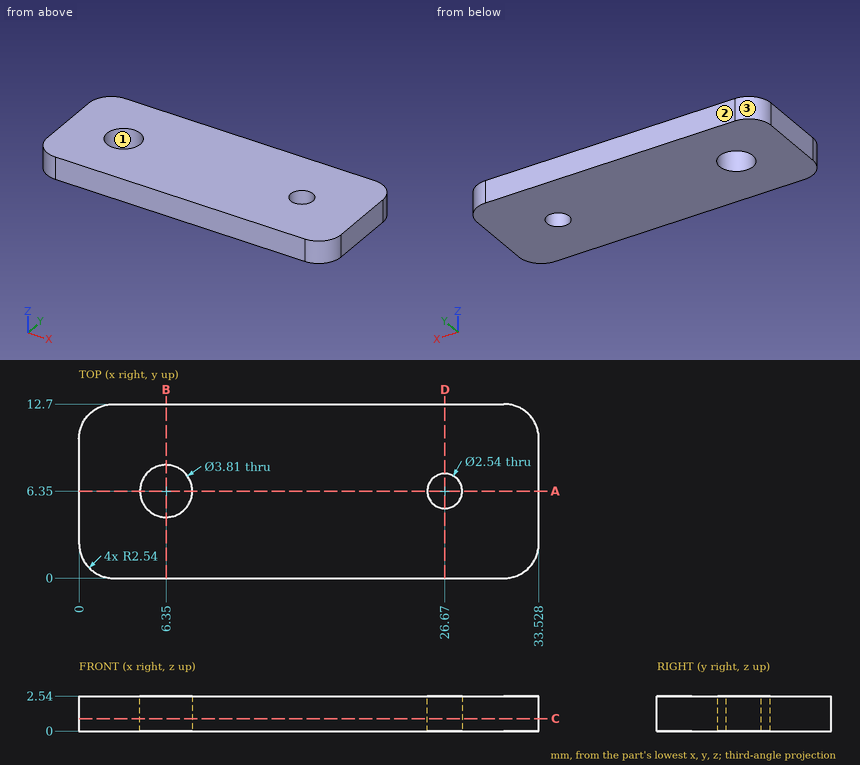
Print and shaded views of the part. All mm, measured from the part's lowest x, y and z. Round coordinates to 2 decimals unless told otherwise and drop trailing zeros. Write each loop counter-clockwise with the first axis right and the second up, starting at its lowest first coordinate (ties: lowest second). Pieces come first, ordered by that corner, then holes.
Item 1: Cut at D-D, the plane x = 26.67. Give the cut face in (y, z).
Results:
outline: (0, 0) - (5.08, 0) - (5.08, 2.54) - (0, 2.54) - close; (7.62, 0) - (12.7, 0) - (12.7, 2.54) - (7.62, 2.54) - close
Item 2: Cut at A-A, the plane y = 6.35. Give the cut face in (x, z) (3 decimals).
Results:
outline: (0, 0) - (4.445, 0) - (4.445, 2.54) - (0, 2.54) - close; (8.255, 0) - (25.4, 0) - (25.4, 2.54) - (8.255, 2.54) - close; (27.94, 0) - (33.528, 0) - (33.528, 2.54) - (27.94, 2.54) - close
Item 3: Cut at B-B, the plane x = 6.35. Give the cut face in (y, z) (3 decimals).
Results:
outline: (0, 0) - (4.445, 0) - (4.445, 2.54) - (0, 2.54) - close; (8.255, 0) - (12.7, 0) - (12.7, 2.54) - (8.255, 2.54) - close
Item 4: Probe L1, parallel to Y at x = 6.35, z = 0.95 (3 decimals); L2, parallel to X at y = 7, z = 2.45; L3, parallel to X at y = 7.75, z = 1.3. List the from-to ranges inside material, lowest first.
Results:
L1: y = 0 to 4.445, 8.255 to 12.7
L2: x = 0 to 4.56, 8.14 to 25.58, 27.76 to 33.53
L3: x = 0 to 5.06, 7.64 to 33.53
Item 5: Drop flat-ended pins along their axis: pin 1 Ø6 at (x, y) = (26, 6) entering from +Z; pin 2 Ø1.5 at (x, y) = (26.67, 6.35) entering from +Z. Give the stop position or say it passes through.
Results:
pin 1: stops at z = 2.54
pin 2: passes through
Item 6: Cut at C-C, the plane z = 0.9. Give the cut face in (x, y) (3 decimals).
Results:
outline: (0, 2.54) arc R2.54 ccw to (2.54, 0) - (30.988, 0) arc R2.54 ccw to (33.528, 2.54) - (33.528, 10.16) arc R2.54 ccw to (30.988, 12.7) - (2.54, 12.7) arc R2.54 ccw to (0, 10.16) - close; hole circle Ø3.81 at (6.35, 6.35); hole circle Ø2.54 at (26.67, 6.35)
Item 7: Two-plate mould, pull along X, no slides. Class the marked faces 1, 2 and 3: +X half, -X half, draft (parallel to the pull), parting line (faces both ways), or undercut.
Results:
face 1: undercut
face 2: draft
face 3: -X half
